Geometry: final body of the model. Coordinates: model frame, mm. A direction names the side the tool comes from. Round coordinates to 2 decimals unless told otherwise and drop trailing zeros. Order: outer loops, then holes, each group sorted by start corner. A loop starts at its lowest first (then second) coordinate and runs counter-clockwise, first axis right, second up. Notation, with made-up numbers: (44, -37) - (96, -37) arc R25 ccw to (96, -21) - close; hole circle Ø4 at (24.25, 47.25). An arc over 180 degrees is marked (long way). Put each result on its own line as item: value. Start each with the question number.
(1) Section A-A (y = 2.5). Output: boundary loops of the cut face in (x, z), and give its area (3 significant figures).
(2) Pull-direction query (X, two-part tool) for faces 1 (the face through (26.458, 7.301, -9.715)), 2 (the face through (28.25, 8.51, 6.08)), 3 (the face through (22.785, 6.699, 0.126)); classes: released by +X, released by -X, zero draft, split by the parting line, or undercut.
(3) Section B-B (x = 26.5). Output: boundary loops of the cut face in (y, z), and give its area (3 significant figures).
(4) Section D-D (z = 2.5). Output: boundary loops of the cut face in (x, y).
(5) Pin query (flat end, axial travel): P1, Ø2, axis at y = 0, z = 0, coming from the +X side; P2, Ø6, axis at x = 7, z = -2, coming from the +Y side; P3, Ø3, axis at x = -26, z = 4.5, coming from the -Y side. Return the tip coordinate at first contact, or that it passes through.
(6) Section C-C (z = 6). Count the separate pieces of the cut face and the enclosed holes in it, and give its area (3 significant figures).
(7) Material intervals for L1, parallel to X at y = 8.3, z = -6; L2, parallel to X at y = 0.75, z = -7.75; L3, parallel to Z at x = -26.5, y = 8.8, sorted ascending. Write a range as [from, to].
(8) Access query for faces 4 (the face through (22.199, 3.535, -9.715)), 5 (the face through (-22.199, 3.465, -9.715)), 6 (the face through (-22.199, 3.535, 9.715)). Directions: +Z, -Z, +X, -X, +Y, -Y. A direction counts if a zero-diameter tool reaches every point of the face in a straight line with its end or side. Return the directions, or none.
from build123d import *

# Parameters (mm, degrees)
F0_W           = 4
F0_H           = 20
F0_W_2         = 37
F1_DEPTH       = 4
F2_DEPTH       = 9
F3_W           = 8
F3_H           = 20
F4_DEPTH       = 2
F6_D           = 3.5
F6_CSINK_D     = 5.5
F6_CSINK_ANGLE = 90
F7_R           = 5
F8_R           = 1


with BuildPart() as f1:
    # F0 (on Front) → F1 (new body)
    with BuildSketch(Plane.XZ):
        with Locations((-20.5, 0)):
            Rectangle(F0_W, F0_H)
        Rectangle(F0_W_2, F0_H)
        with Locations((20.5, 0)):
            Rectangle(F0_W, F0_H)
    extrude(amount=F1_DEPTH)

    # F0 (on Front) → F2 (join)
    with BuildSketch(Plane.XZ):
        with Locations((-20.5, 0)):
            Rectangle(F0_W, F0_H)
        with Locations((20.5, 0)):
            Rectangle(F0_W, F0_H)
    extrude(amount=-F2_DEPTH)

    # F3 (on face) → F4 (join)
    with BuildSketch(Plane(origin=(0, 9, 0), x_dir=(-1, 0, 0), z_dir=(0, 1, 0))):
        with Locations((-26.5, 0)):
            Rectangle(F3_W, F3_H)
        with Locations((26.5, 0)):
            Rectangle(F3_W, F3_H)
    extrude(amount=-F4_DEPTH)

    # F6 (through all)
    with Locations(Plane.XZ.offset(-7)):
        with Locations((-26.5, -6), (-26.5, 6), (26.5, -6), (26.5, 6)):
            CounterSinkHole(F6_D / 2, F6_CSINK_D / 2, counter_sink_angle=F6_CSINK_ANGLE)

    # F7
    f7_edges = [f1.edges().sort_by_distance(p)[0] for p in [
        (22.5, -4, 0),
        (-22.5, -4, 0),
    ]]
    fillet(f7_edges, radius=F7_R)

    # F8
    f8_edges = [f1.edges().sort_by_distance(p)[0] for p in [
        (22.5, 7, 0),
        (-22.5, 7, 0),
        (26.5, 7, 10),
        (26.5, 7, -10),
        (30.5, 7, 0),
        (-30.5, 7, 0),
        (30.5, 8, 10),
        (30.5, 8, -10),
        (-30.5, 8, 10),
        (-30.5, 8, -10),
        (-22.5, 4, -10),
        (-21.035534, -2.535534, -10),
        (-26.5, 7, -10),
        (0, -4, -10),
        (21.035534, -2.535534, -10),
        (22.5, 4, -10),
        (-22.5, 4, 10),
        (-21.035534, -2.535534, 10),
        (-26.5, 7, 10),
        (0, -4, 10),
        (21.035534, -2.535534, 10),
        (22.5, 4, 10),
    ]]
    fillet(f8_edges, radius=F8_R)


solid = f1.part
Checks:
1. outline: (-22.5, -9) arc R1 ccw to (-21.5, -10) - (-18.5, -10) - (-18.5, 10) - (-21.5, 10) arc R1 ccw to (-22.5, 9) - close; (18.5, -10) - (21.5, -10) arc R1 ccw to (22.5, -9) - (22.5, 9) arc R1 ccw to (21.5, 10) - (18.5, 10) - close
1. area: 159 mm²
2. face 1: zero draft
2. face 2: undercut
2. face 3: released by +X
3. outline: (7, -9) arc R1 ccw to (8, -10) - (9, -10) - (9, -7.75) - (8, -7.75) - (7, -8.75) - close; (7, -3.25) - (8, -4.25) - (9, -4.25) - (9, 4.25) - (8, 4.25) - (7, 3.25) - close; (7, 8.75) - (8, 7.75) - (9, 7.75) - (9, 10) - (8, 10) arc R1 ccw to (7, 9) - close
3. area: 23.6 mm²
4. outline: (-30.5, 8) arc R1 ccw to (-29.5, 7) - (-23.5, 7) arc R1 cw to (-22.5, 6) - (-22.5, 1) arc R5 ccw to (-17.5, -4) - (17.5, -4) arc R5 ccw to (22.5, 1) - (22.5, 6) arc R1 cw to (23.5, 7) - (29.5, 7) arc R1 ccw to (30.5, 8) - (30.5, 9) - (18.5, 9) - (18.5, 0) - (-18.5, 0) - (-18.5, 9) - (-30.5, 9) - close
5. P1: stops at x = 22.5
5. P2: stops at y = 0
5. P3: stops at y = 7
6. separate pieces: 3
6. enclosed holes: 0
6. area: 257 mm²
7. L1: x = [-30.5, -28.25], [-24.75, -18.5], [18.5, 24.75], [28.25, 30.5]
7. L2: x = [-22.49, -18.5], [18.5, 22.49]
7. L3: z = [-10, -7.75], [-4.25, 4.25], [7.75, 10]
8. face 4: -Z, +X, -Y
8. face 5: -Z, -X, -Y
8. face 6: +Z, -X, -Y
